Read the model definition and answer for the solid it produces. Units are mm, in the model's axes. Round coordinates to 2 decimals unless told otherwise and drop trailing zeros. Write each loop counter-clockwise with the first axis right and the second up, starting at its lowest first coordinate (ties: lowest second). Pieces come first, ordered by that corner, then holes.
from build123d import *

# Parameters (mm, degrees)
SKETCH_1_W          = 500.8
SKETCH_1_H          = 300.8
EXTRUDE_1_DEPTH     = 4.75
SKETCH_2_W          = 25.4
SKETCH_2_H          = 25.4
SKETCH_2_W_2        = 4.75
SKETCH_2_H_2        = 80
CUT_EXTRUDE_1_DEPTH = 25.4
SKETCH_3_R          = 2.15
SKETCH_3_R_2        = 2.150000004
CUT_EXTRUDE_2_DEPTH = 5
SKETCH_5_W          = 35
SKETCH_5_H          = 60
SKETCH_5_W_2        = 300
SKETCH_5_H_2        = 30
CUT_EXTRUDE_3_DEPTH = 10
FILLET_1_R          = 7
SKETCH_6_R          = 1.75
CUT_EXTRUDE_4_DEPTH = 10


with BuildPart() as part:
    # 草圖1 → 填料-伸長1 (new body)
    with BuildSketch(Plane.XY):
        Rectangle(SKETCH_1_W, SKETCH_1_H)
    extrude(amount=EXTRUDE_1_DEPTH)

    # 草圖2 → 除料-伸長1 (cut)
    with BuildSketch(Plane(origin=(0, 0, 0), x_dir=(-1, 0, 0), z_dir=(0, 0, -1))):
        with Locations((-237.7, 137.7)):
            Rectangle(SKETCH_2_W, SKETCH_2_H)
        with Locations((-237.7, -137.7)):
            Rectangle(SKETCH_2_W, SKETCH_2_H)
        with Locations((237.7, 137.7)):
            Rectangle(SKETCH_2_W, SKETCH_2_H)
        with Locations((237.7, -137.7)):
            Rectangle(SKETCH_2_W, SKETCH_2_H)
        with Locations((-222.625, 65.4)):
            Rectangle(SKETCH_2_W_2, SKETCH_2_H_2)
        with Locations((-222.625, -65.4)):
            Rectangle(SKETCH_2_W_2, SKETCH_2_H_2)
        with Locations((222.625, 65.4)):
            Rectangle(SKETCH_2_W_2, SKETCH_2_H_2)
        with Locations((222.625, -64.4)):
            Rectangle(SKETCH_2_W_2, SKETCH_2_H_2)
        with Locations((-72.625, 65.4)):
            Rectangle(SKETCH_2_W_2, SKETCH_2_H_2)
        with Locations((77.375, 65.4)):
            Rectangle(SKETCH_2_W_2, SKETCH_2_H_2)
        with Locations((77.375, -65.4)):
            Rectangle(SKETCH_2_W_2, SKETCH_2_H_2)
        with Locations((-72.625, -65.4)):
            Rectangle(SKETCH_2_W_2, SKETCH_2_H_2)
    extrude(amount=-CUT_EXTRUDE_1_DEPTH, mode=Mode.SUBTRACT)

    # 草圖3 → 除料-伸長2 (cut)
    with BuildSketch(Plane.XY.offset(4.75)):
        with Locations((-207.3, 137.7)):
            Circle(SKETCH_3_R)
        with Locations((-182.8, 137.7)):
            Circle(SKETCH_3_R)
        with Locations((182.8, 137.7)):
            Circle(SKETCH_3_R)
        with Locations((207.3, 137.7)):
            Circle(SKETCH_3_R)
        with Locations((237.7, 107.3)):
            Circle(SKETCH_3_R)
        with Locations((237.7, 82.8)):
            Circle(SKETCH_3_R)
        with Locations((237.7, -82.800000014)):
            Circle(SKETCH_3_R_2)
        with Locations((237.7, -107.300000014)):
            Circle(SKETCH_3_R_2)
        with Locations((-237.7, 107.3)):
            Circle(SKETCH_3_R)
        with Locations((-237.7, 82.8)):
            Circle(SKETCH_3_R)
        with Locations((-237.7, -82.800000014)):
            Circle(SKETCH_3_R_2)
        with Locations((-237.7, -107.300000014)):
            Circle(SKETCH_3_R_2)
    extrude(amount=-CUT_EXTRUDE_2_DEPTH, mode=Mode.SUBTRACT)

    # 草圖5 → 除料-伸長3 (cut)
    with BuildSketch(Plane.XY.offset(4.75)):
        with Locations((100, -65.4)):
            Rectangle(SKETCH_5_W, SKETCH_5_H)
        with Locations((-50, -65.4)):
            Rectangle(SKETCH_5_W, SKETCH_5_H)
        with Locations((-195.25, -65.4)):
            Rectangle(SKETCH_5_W, SKETCH_5_H)
        with Locations((0, 135.4)):
            Rectangle(SKETCH_5_W_2, SKETCH_5_H_2)
    extrude(amount=-CUT_EXTRUDE_3_DEPTH, mode=Mode.SUBTRACT)

    # 圓角1
    fillet_1_edges = [part.edges().sort_by_distance(p)[0] for p in [
        (-150, 120.4, 2.375),
        (150, 120.4, 2.375),
        (-177.75, -35.4, 2.375),
        (-177.75, -95.4, 2.375),
        (-212.75, -95.4, 2.375),
        (-212.75, -35.4, 2.375),
        (-32.5, -35.4, 2.375),
        (-32.5, -95.4, 2.375),
        (-67.5, -95.4, 2.375),
        (-67.5, -35.4, 2.375),
        (117.5, -35.4, 2.375),
        (117.5, -95.4, 2.375),
        (82.5, -95.4, 2.375),
        (82.5, -35.4, 2.375),
    ]]
    fillet(fillet_1_edges, radius=FILLET_1_R)

    # 草圖6 → 除料-伸長4 (cut)
    with BuildSketch(Plane.XY.offset(4.75)):
        with Locations((-202.75, -142.9)):
            Circle(SKETCH_6_R)
        with Locations((-202.75, -123.9)):
            Circle(SKETCH_6_R)
        with Locations((-57.5, -142.9)):
            Circle(SKETCH_6_R)
        with Locations((-57.5, -123.9)):
            Circle(SKETCH_6_R)
        with Locations((87.75, -142.9)):
            Circle(SKETCH_6_R)
        with Locations((87.75, -123.9)):
            Circle(SKETCH_6_R)
    extrude(amount=-CUT_EXTRUDE_4_DEPTH, mode=Mode.SUBTRACT)


solid = part.part
Q1. Flat-ended cylindrical pins translate along their axes: pin 1 Ø2.5 at (x, y) = (-237.7, -107.3) entering from +Z; pin 2 Ø1.5 at (x, z) = (-9, 0.5) entering from +Y; pin 3 Ø1.4 at (x, z) = (244, 3) entering from +Y. Find the tip coordinate at first contact, or state that the pin passes through.
Verdict:
pin 1: passes through
pin 2: stops at y = 120.4
pin 3: stops at y = 125
Q2. Section C-C (z = 0.9) is taken. State how many separate pieces and enclosed holes the cut face has, then the cut area to 3 significant figures.
Verdict:
separate pieces: 1
enclosed holes: 29
area: 130,000 mm2
Q3. Section B-B (x = 137) is taken. Determine the outline of the cut face in (y, z), then the cut area to 3 significant figures.
Verdict:
outline: (-150.4, 0) - (120.4, 0) - (120.4, 4.75) - (-150.4, 4.75) - close
area: 1,290 mm2
Q4. Section A-A (y = 73) is taken. Determine the outline of the cut face in (x, z), then the cut area to 3 significant figures.
Verdict:
outline: (-250.4, 0) - (-225, 0) - (-225, 4.75) - (-250.4, 4.75) - close; (-220.25, 0) - (-79.75, 0) - (-79.75, 4.75) - (-220.25, 4.75) - close; (-75, 0) - (70.25, 0) - (70.25, 4.75) - (-75, 4.75) - close; (75, 0) - (220.25, 0) - (220.25, 4.75) - (75, 4.75) - close; (225, 0) - (250.4, 0) - (250.4, 4.75) - (225, 4.75) - close
area: 2,290 mm2
Q5. Straight lines are drawn through the part: probe 1 along X at (y, z) = (89, 1.65); probe 2 along Y at (x, z) = (-202.75, 2.55); probe 3 along X at (y, z) = (-104.5, 2.3). For each, find the intervals that lie inside material, in ascending order.
Verdict:
probe 1: x = -250.4 to -225, -220.25 to -79.75, -75 to 70.25, 75 to 220.25, 225 to 250.4
probe 2: y = -150.4 to -144.65, -141.15 to -125.65, -122.15 to -95.4, -35.4 to 150.4
probe 3: x = -250.4 to -79.75, -75 to 70.25, 75 to 220.25, 225 to 250.4
